```python
from build123d import *

# Parameters (mm, degrees)
SALIENTE_EXTRUIR1_DEPTH = 28
CROQUIS2_R              = 4.25
CORTAR_EXTRUIR1_DEPTH   = 25
CORTAR_EXTRUIR2_REACH   = 42.1
CROQUIS3_R              = 1.7
SALIENTE_EXTRUIR2_DEPTH = 1.2
REDONDEO1_R             = 2


with BuildPart() as part:
    # Croquis1 → Saliente-Extruir1 (new body)
    with BuildSketch(Plane.XY):
        Polygon((0, 4.2), (-14, 4.2), (-14, 40.1), (-24, 40.1), (-24, 0), (0, 0), align=None)
    extrude(amount=SALIENTE_EXTRUIR1_DEPTH)

    # Croquis2 → Cortar-Extruir1 (cut, through all)
    with BuildSketch(Plane.ZY.offset(24)):
        with Locations((10, 30.1)):
            Circle(CROQUIS2_R)
        with BuildLine():
            Line((28, 5), (19.575461286, 32.982800922))
            ThreePointArc((19.575461286, 32.982800922), (8.54305334, 39.993296035), (0, 30.1))
            Line((0, 30.1), (0, 29.1))
            Line((0, 29.1), (-1, 29.1))
            Line((-1, 29.1), (-1, 41.1))
            Line((-1, 41.1), (29, 41.1))
            Line((29, 41.1), (29, 5))
            Line((29, 5), (28, 5))
        make_face()
    extrude(amount=-CORTAR_EXTRUIR1_DEPTH, mode=Mode.SUBTRACT)

    # Croquis3 → Cortar-Extruir2 (cut, up to next)
    with BuildSketch(Plane.XZ, mode=Mode.PRIVATE) as cortar_extruir2_sk1:
        with Locations((-9, 22)):
            Circle(CROQUIS3_R)
    cortar_extruir2_tool1 = extrude(cortar_extruir2_sk1.sketch, amount=-CORTAR_EXTRUIR2_REACH, mode=Mode.PRIVATE) & part.part
    add(cortar_extruir2_tool1.solids().sort_by_distance((-9, 0, 22))[0], mode=Mode.SUBTRACT)
    # Croquis3 → Cortar-Extruir2 (cut, up to next)
    with BuildSketch(Plane.XZ, mode=Mode.PRIVATE) as cortar_extruir2_sk2:
        with Locations((-9, 6)):
            Circle(CROQUIS3_R)
    cortar_extruir2_tool2 = extrude(cortar_extruir2_sk2.sketch, amount=-CORTAR_EXTRUIR2_REACH, mode=Mode.PRIVATE) & part.part
    add(cortar_extruir2_tool2.solids().sort_by_distance((-9, 0, 6))[0], mode=Mode.SUBTRACT)

    # Croquis4 → Saliente-Extruir2 (add, symmetric)
    with BuildSketch(Plane(origin=(0, 0, 14), x_dir=(-1, 0, 0), z_dir=(0, 0, -1))):
        Polygon((0, 4.2), (14, 4.2), (14, 20.2), (12, 20.2), (0, 6.3), align=None)
    extrude(amount=SALIENTE_EXTRUIR2_DEPTH, both=True)

    # Redondeo1
    redondeo1_edges = [part.edges().sort_by_distance(p)[0] for p in [
        (-7, 4.2, 15.2),
        (-7, 4.2, 12.8),
    ]]
    fillet(redondeo1_edges, radius=REDONDEO1_R)


solid = part.part
```
Verification items for the finished model (mm, model axes). A direction names the side the tool comes from. Give positions to 0.01 mm unless a question says otherwise; leave off trailing zeros. Order: outer loops, then holes, each group sorted by start corner. A loop starts at its lowest first (then second) coordinate and runs counter-clockwise, first axis right, second up. Notation, with made-up numbers: M 14,10 L 52,10 A21 cw 52,38 Z; hole C 14.5,-3 d8. An arc over 180 degrees is marked long. Answer in a Markdown table with one row per item. Add a question column.
Item 1: Gauge pin test, flat ends, axial feed: pin 1 (8 mm diameter, centred on x = -18.5, z = 9.5, fed in from +Y); pin 2 (8.5 mm diameter, centred on x = -8, z = 24.5, fed in from +Y); pin 3 (3 mm diameter, centred on x = -6, z = 14, fed in from +Y); pin 4 (1 mm diameter, centred on y = 25.5, z = 3, fed in from +X). Record the tip position at first contact, or that the pin passes through.
Item 2: Tool access check on faces 4 (the flat face through (-7, 4.2, 23)), 5 (the flat face through (-13, 20.2, 14)), 6 (the flat face through (-19.07, 18.796, 23.847)), 7 (the flat face through (-8, 12, 12.8)). Record the directions out of +Z, -Z, +X, -X, +Y, -Y that give a thin tool (end or side, any length) a straight path to the whole face; none if there is none.
Item 3: Scan lines: probe 1 along Z at (x, y) = (-9, 2.3); probe 2 along Y at (x, z) = (-21.5, 10); probe 3 along Y at (x, z) = (-1.5, 9). Record each from-to range of solid material in increasing order. Write a range as from..to.
Item 4: Section check B-B, the plane z = 11.75. Enter the section's corners in (x, y).
Item 5: Section check A-A, the plane x = -21.5. Enter the section's corners in (y, z).
Item 6: Mould release check, pull along Z, two halves, no side actions. Record for faces 1 (the cylindrical face through (-7.1, 4.77, 12.2)), 2 (the cylindrical face through (-19.07, 40.02, 8.74)), 3 (the cylindrical face through (-9.37, 2.07, 4.34)): released by +Z, released by -Z, zero draft, split by the parting line, or undercut.
Item 7: Section check C-C, the plane x = -9. Enter the section's corners in (y, z) (3 decimals).
Item 8: Section check D-D, the plane y = 32. Enter the section's corners in (x, z), and give its area (3 significant figures).
Filled sheet:
| question | item | result |
|---|---|---|
| 1 | pin 1 | stops at y = 40.1 |
| 1 | pin 2 | stops at y = 4.2 |
| 1 | pin 3 | stops at y = 14.99 |
| 1 | pin 4 | stops at x = -14 |
| 2 | face 4 | +Z, +X, +Y |
| 2 | face 5 | +Z, -Z, +X, +Y |
| 2 | face 6 | +Z, +X, -X, +Y |
| 2 | face 7 | -Z, +X, +Y |
| 3 | probe 1 | z = 0..4.3, 7.7..20.3, 23.7..28 |
| 3 | probe 2 | y = 0..25.85, 34.35..40.1 |
| 3 | probe 3 | y = 0..4.2 |
| 4 | outline | M -24,0 L 0,0 L 0,4.44 L -14,4.44 L -14,26.23 L -24,26.23 Z; M -24,33.97 L -14,33.97 L -14,39.95 L -24,39.95 Z |
| 5 | outline | M 0,0 L 30.1,0 A10 ccw 32.98,19.58 L 5,28 L 0,28 Z; hole C 30.1,10 d8.5 |
| 6 | face 1 | released by -Z |
| 6 | face 2 | split by the parting line |
| 6 | face 3 | undercut |
| 7 | outline | M 0,0 L 4.2,0 L 4.2,4.3 L 0,4.3 Z; M 0,7.7 L 4.2,7.7 L 4.2,10.8 A2 cw 6.2,12.8 L 16.725,12.8 L 16.725,15.2 L 6.2,15.2 A2 cw 4.2,17.2 L 4.2,20.3 L 0,20.3 Z; M 0,23.7 L 4.2,23.7 L 4.2,28 L 0,28 Z |
| 8 | outline | M -24,0.18 L -14,0.18 L -14,6.2 L -24,6.2 Z; M -24,13.8 L -14,13.8 L -14,19.87 L -24,19.87 Z |
| 8 | area | 121 mm^2 |
